from build123d import *

# Parameters (mm, degrees)
SKETCH_R     = 1.5
SKETCH_R_2   = 10.5
PAD_DEPTH    = 3
SKETCH001_W  = 5.5
SKETCH001_H  = 20
POCKET_DEPTH = 3.001


with BuildPart() as part:
    # Sketch → Pad (new body)
    with BuildSketch(Plane.XY):
        with BuildLine():
            ThreePointArc((-16, 0), (0, -16), (16, 0))
            Line((16, 50), (16, 0))
            Line((-16, 50), (16, 50))
            Line((-16, 0), (-16, 50))
        make_face()
        with Locations((0, 12.6)):
            Circle(SKETCH_R, mode=Mode.SUBTRACT)
        with Locations((10.91192, -6.3)):
            Circle(SKETCH_R, mode=Mode.SUBTRACT)
        with Locations((-10.91192, -6.3)):
            Circle(SKETCH_R, mode=Mode.SUBTRACT)
        Circle(SKETCH_R_2, mode=Mode.SUBTRACT)
        with Locations((-4.5, 45)):
            Circle(SKETCH_R, mode=Mode.SUBTRACT)
        with Locations((4.5, 45)):
            Circle(SKETCH_R, mode=Mode.SUBTRACT)
        with Locations((-4.5, 25)):
            Circle(SKETCH_R, mode=Mode.SUBTRACT)
        with Locations((4.5, 25)):
            Circle(SKETCH_R, mode=Mode.SUBTRACT)
    extrude(amount=PAD_DEPTH)

    # Sketch001 → Pocket (cut, through all)
    with BuildSketch(Plane.XY.offset(3)):
        with Locations((-13.25, 40)):
            Rectangle(SKETCH001_W, SKETCH001_H)
        with Locations((13.25, 40)):
            Rectangle(SKETCH001_W, SKETCH001_H)
    extrude(amount=-POCKET_DEPTH, mode=Mode.SUBTRACT)


solid = part.part
Here's how the part is built. I have some questions about the finished solid (model axes, mm). A direction names the side the tool comes from. Give positions to 0.01 mm unless a question says otherwise; leave off trailing zeros. Loops run counter-clockwise (first coordinate to the right, second up) from the corner with the lowest first, then second, coordinate; pieces in that order, holes last. Notation, with made-up numbers: (65.5, 27) -> (95.5, 27) arc R14 ccw to (95.5, 36) -> close; hole circle Ø3 at (25, 26.5). An arc over 180 degrees is marked (long way). Answer as a JSON object with one key per item and string values. Group by question number.
Item 1: Will these pins go through, and if not, where does the flat tip stop? pin 1 (1.5 mm diameter, centred on x = -12, z = 2, fed in from +Y); pin 2 (1 mm diameter, centred on x = 10.5, z = 2.5, fed in from -Y).
Item 2: Thinking about a two-plate mould opening in Y: for faces 4 (the cylindrical face through (0, -16, 1)), 5 (the flat face through (16, 15, 1)), 6 (the cylindrical face through (-4.825, 43.536, 1.479)), which applies, pulls with the +Y half, pulls with the -Y half, needs draft (parallel to the pull), parting line crosses it, or undercut?
Item 3: Imagine slicing it at B-B on z = 0.5. Give the number of separate pieces and of enclosed holes in the cut face, then the cut area to 3 significant figures.
Item 4: Imagine slicing it at A-A on y = 12.6. Write out the boundary of the cut face in (x, z), then the cut area to 3 significant figures.
Item 5: On a 3-axis mill with a long thin cutter (end or side, diameter ignored), from which of +Z, -Z, +X, -X, +Y, -Y can I reach the whole of each face in a straight line? I mean faces 1 (the flat face through (10.5, 40, 2)), 2 (the cylindrical face through (11.604, -7.631, 1.479)), 3 (the flat face through (-13, 30, 2)). Say none if no direction works.
Item 6: Imagine slicing it at D-D on x = 0. Write out the boundary of the cut face in (y, z).
Item 7: I need wall thicknesses on L1, parallel to Y at x = 0, z = 2.4; L2, parallel to X at y = -6.5, z = 1.9; L3, parallel to Y at x = 5, z = 2.65. Which ranges of each line are inside material? Lowest first, please.
Item 8: Imagine slicing it at C-C on y = 25. Write out the boundary of the cut face in (x, z).
Answer list:
{
 "1": {"pin 1": "stops at y = 30", "pin 2": "stops at y = -12.49"},
 "2": {"face 4": "pulls with the -Y half", "face 5": "needs draft", "face 6": "undercut"},
 "3": {"separate pieces": "1", "enclosed holes": "8", "area": "1,390 mm2"},
 "4": {"outline": "(-16, 0) -> (-1.5, 0) -> (-1.5, 3) -> (-16, 3) -> close; (1.5, 0) -> (16, 0) -> (16, 3) -> (1.5, 3) -> close", "area": "87.0 mm2"},
 "5": {"face 1": "+Z, -Z, +X, +Y", "face 2": "+Z, -Z", "face 3": "+Z, -Z, -X, +Y"},
 "6": {"outline": "(-16, 0) -> (-10.5, 0) -> (-10.5, 3) -> (-16, 3) -> close; (10.5, 0) -> (11.1, 0) -> (11.1, 3) -> (10.5, 3) -> close; (14.1, 0) -> (50, 0) -> (50, 3) -> (14.1, 3) -> close"},
 "7": {"L1": "y = -16 to -10.5, 10.5 to 11.1, 14.1 to 50", "L2": "x = -14.62 to -12.4, -9.43 to -8.25, 8.25 to 9.43, 12.4 to 14.62", "L3": "y = -15.2 to -9.23, 9.23 to 23.59, 26.41 to 43.59, 46.41 to 50"},
 "8": {"outline": "(-16, 0) -> (-6, 0) -> (-6, 3) -> (-16, 3) -> close; (-3, 0) -> (3, 0) -> (3, 3) -> (-3, 3) -> close; (6, 0) -> (16, 0) -> (16, 3) -> (6, 3) -> close"}
}
